Source: CAD feature listing. Evaluate the final solid. Frame: model axes, mm. A direction names the side the tool comes from. Give positions to 0.01 mm unless a question says otherwise; leave off trailing zeros. Order: outer loops, then holes, each group sorted by start corner. A loop starts at its lowest first (then second) coordinate and runs counter-clockwise, first axis right, second up. Notation, with made-up numbers: M 80,36.25 L 89,36.25 A22 ccw 89,58.25 Z; hole C 37.25,-20 d4. An arc over 180 degrees is marked long. Use CSV: the item, a comma, the result in double quotes. Start each with the question number.
Item 1: First-contact query: pin 1 (1.5 mm diameter, centred on x = 4, y = -8, fed in from +Z); pin 2 (5 mm diameter, centred on y = -7.5, z = -14.5, fed in from +X); pin 3 (14.5 mm diameter, centred on y = 0, z = 0, fed in from +X); pin 4 (5 mm diameter, centred on y = 3, z = 1.5, fed in from -X). Flat tips, straight axial feed; report the tip coordinate or a pass-through.
Item 2: Ray query, probe 1 along Y at (x, z) = (8.3, 0); probe 2 along X at (y, z) = (14.5, -3.5); probe 3 along Y at (x, z) = (8.25, 14.5). Return the intervals inside material, ascending. Write a range as from..to.
Item 3: Pull-direction query (Y, two-part tool) for faces 1 (the face through (10, -8.2, 0.2)), 2 (the face through (4.93, -15.821, 20.633)), 3 (the face through (4.25, 7, 0)); classes: +Y half, -Y half, draft (parallel to the pull), parting line (faces both ways), or undercut.
Item 4: Section query D-D on y = -17. Return loops of the section in (x, z), and give its area (3 significant figures).
Item 5: Section query A-A on x = 1.5. Return loops of the section in (y, z), and give its area (3 significant figures).
Item 6: Access query for faces 4 (the face through (10, 19.4, 11.7)), 5 (the face through (1.479, 3.755, -11.923)), 6 (the face through (7.85, -7.81, 1.73)). Directions: +Z, -Z, +X, -X, +Y, -Y. A direction counts if a zero-diameter tool reaches every point of the face in a straight line with its end or side. Return the directions, or none.
from build123d import *

# Parameters (mm, degrees)
SKETCH1_R           = 26
SKETCH1_R_2         = 8
BOSS_EXTRUDE1_DEPTH = 10
SKETCH2_R           = 8
SKETCH2_R_2         = 6.5
BOSS_EXTRUDE2_DEPTH = 0.75
SKETCH3_R           = 22.5
SKETCH3_R_2         = 12.5
CUT_EXTRUDE1_DEPTH  = 3


with BuildPart() as part:
    # Sketch1 → Boss-Extrude1 (new body)
    with BuildSketch(Plane(origin=(0, 0, 0), x_dir=(0, 0, -1), z_dir=(1, 0, 0))):
        Circle(SKETCH1_R)
        Circle(SKETCH1_R_2, mode=Mode.SUBTRACT)
    extrude(amount=BOSS_EXTRUDE1_DEPTH)

    # Sketch2 → Boss-Extrude2 (add, symmetric)
    with BuildSketch(Plane(origin=(5, 0, 0), x_dir=(0, 0, -1), z_dir=(1, 0, 0))):
        Circle(SKETCH2_R)
        Circle(SKETCH2_R_2, mode=Mode.SUBTRACT)
    extrude(amount=BOSS_EXTRUDE2_DEPTH, both=True)

    # Sketch3 → Cut-Extrude1 (cut)
    with BuildSketch(Plane(origin=(10, 0, 0), x_dir=(0, 0, -1), z_dir=(1, 0, 0))):
        Circle(SKETCH3_R)
        Circle(SKETCH3_R_2, mode=Mode.SUBTRACT)
    cut_extrude1 = extrude(amount=-CUT_EXTRUDE1_DEPTH, mode=Mode.SUBTRACT)

    # Mirror1: Cut-Extrude1 across plane
    add(cut_extrude1.mirror(Plane(origin=(5, 0, 0), x_dir=(0, 0, 1), z_dir=(1, 0, 0))), mode=Mode.SUBTRACT)


solid = part.part
Verdict:
1,pin 1,"z = 24.97"
1,pin 2,"x = 7"
1,pin 3,"x = 5.75"
1,pin 4,"through"
2,probe 1,"-26..-22.5, -12.5..-8, 8..12.5, 22.5..26"
2,probe 2,"3..7"
2,probe 3,"-21.58..-17.2, 17.2..21.58"
3,face 1,"draft"
3,face 2,"parting line"
3,face 3,"undercut"
4,outline,"M 0,-19.67 L 10,-19.67 L 10,-14.74 L 7,-14.74 L 7,14.74 L 10,14.74 L 10,19.67 L 0,19.67 L 0,14.74 L 3,14.74 L 3,-14.74 L 0,-14.74 Z"
4,area,"217 mm2"
5,outline,"C 0,0 d52; C 0,0 d25; hole C 0,0 d45; hole C 0,0 d16"
5,area,"823 mm2"
6,face 4,"+Z, -Z, +X, +Y, -Y"
6,face 5,"-X"
6,face 6,"+X"
